Source: three-view drawing plus pictorial views. Frame: mm from the lowest corner of the part. A direction names the side the tool comes from. Round coordinates to 2 decimals unless told otherwise and drop trailing zeros. Order: outer loops, then holes, each group sorted by start corner. A loop starts at its lowest first (then second) coordinate and runs counter-clockwise, first axis right, second up. Notation, with made-up numbers: (0, -38) - (5, -38) arc R20 cw to (5, -5) - close; hole circle Ø7 at (-38, -11.75). An arc over 180 degrees is marked (long way). One line per item, written item: value. Start each with the question number.
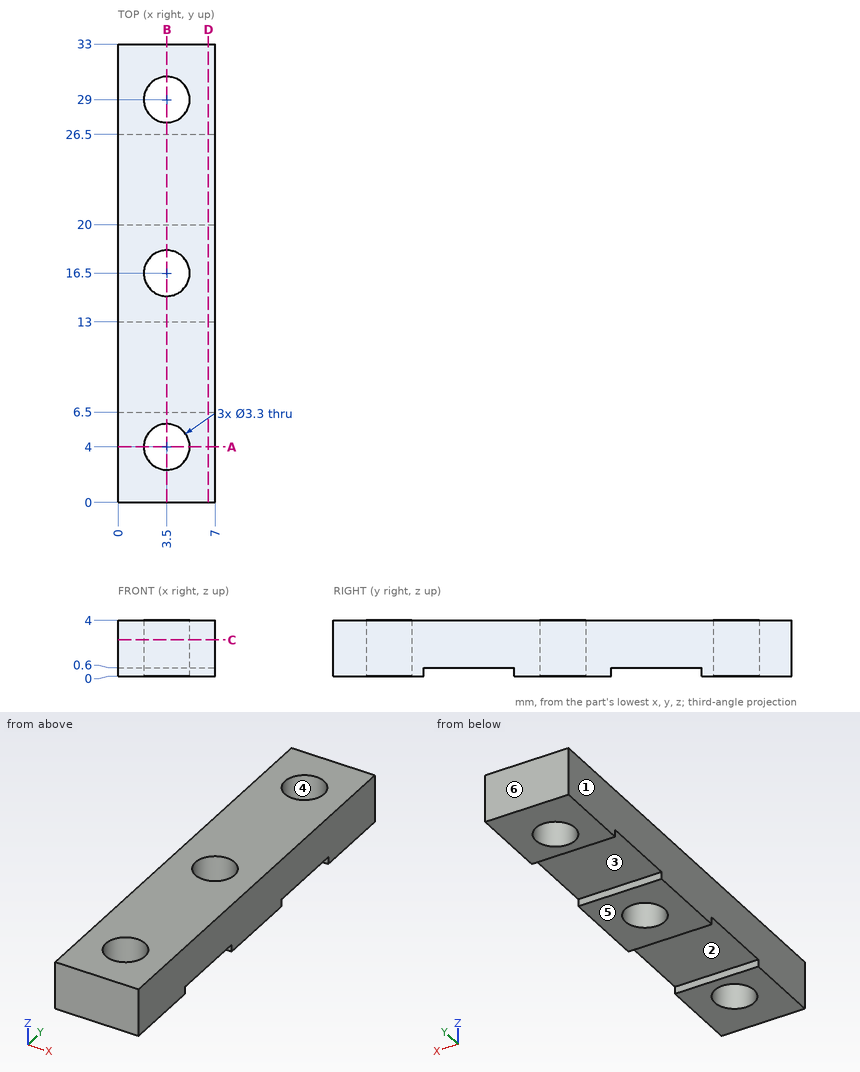
Item 1: Section query A-A on y = 4. Return loops of the section in (x, z).
Item 2: Section query D-D on x = 6.5. Return loops of the section in (y, z).
Item 3: Section query B-B on x = 3.5. Return loops of the section in (y, z), and give its area (3 significant figures).
Item 4: Pull-direction query (Y, two-part tool) for the marked faces 3, 4, 5 and 6; classes: released by +Y, released by -Y, zero draft, split by the parting line, or undercut.
Item 5: Reachability of the marked faces 1 and 2 from +Z, -Z, +X, -X, +Y, -Y: full face, straight path, thin tool, end or side. Return the list, or none.
Item 6: Line query: L1, parallel to Y at x = 3.5, z = 2.85; L2, parallel to Y at x = 2.5, z = 3.5; L3, parallel to Y at x = 4.5, z = 0.55. Output: solid intervals per line, ascending.
Item 7: Section query C-C on z = 2.6. Return loops of the section in (x, y), and give its area (3 significant figures).
Item 8: First-contact query: pin 1 Ø2 at (x, y) = (3.5, 29) entering from -Z; pin 2 Ø2 at (x, y) = (4.5, 24) entering from -Z. Flat tips, straight axial feed; report the tip coordinate or a pass-through.
Geometry results:
1. outline: (0, 0) - (1.85, 0) - (1.85, 4) - (0, 4) - close; (5.15, 0) - (7, 0) - (7, 4) - (5.15, 4) - close
2. outline: (0, 0) - (6.5, 0) - (6.5, 0.6) - (13, 0.6) - (13, 0) - (20, 0) - (20, 0.6) - (26.5, 0.6) - (26.5, 0) - (33, 0) - (33, 4) - (0, 4) - close
3. outline: (0, 0) - (2.35, 0) - (2.35, 4) - (0, 4) - close; (5.65, 0) - (6.5, 0) - (6.5, 0.6) - (13, 0.6) - (13, 0) - (14.85, 0) - (14.85, 4) - (5.65, 4) - close; (18.15, 0) - (20, 0) - (20, 0.6) - (26.5, 0.6) - (26.5, 0) - (27.35, 0) - (27.35, 4) - (18.15, 4) - close; (30.65, 0) - (33, 0) - (33, 4) - (30.65, 4) - close
3. area: 84.6 mm^2
4. face 3: undercut
4. face 4: undercut
4. face 5: zero draft
4. face 6: released by +Y
5. face 1: +Z, -Z, -X, +Y, -Y
5. face 2: -Z, +X, -X
6. L1: y = 0 to 2.35, 5.65 to 14.85, 18.15 to 27.35, 30.65 to 33
6. L2: y = 0 to 2.69, 5.31 to 15.19, 17.81 to 27.69, 30.31 to 33
6. L3: y = 0 to 2.69, 5.31 to 6.5, 13 to 15.19, 17.81 to 20, 26.5 to 27.69, 30.31 to 33
7. outline: (0, 0) - (7, 0) - (7, 33) - (0, 33) - close; hole circle Ø3.3 at (3.5, 4); hole circle Ø3.3 at (3.5, 16.5); hole circle Ø3.3 at (3.5, 29)
7. area: 205 mm^2
8. pin 1: passes through
8. pin 2: stops at z = 0.6
